For this review, take the finished solid that the model builds, in its own axes (mm). A direction names the side the tool comes from. Give positions to 0.01 mm unless a question says otherwise; leave off trailing zeros. Loops run counter-clockwise (first coordinate to the right, second up) from the corner with the lowest first, then second, coordinate; pieces in that order, holes last. Notation, with made-up numbers: M -1,-1 L 21,-1 A26 cw 21,25 Z; hole C -33,25 d2. An arc over 180 degrees is marked long. Use CSV: the item, a comma, the result in double quotes. Start each with the question number.
1. Take a section at D-D, the plane y = 19.5. Write out the cut boundary in (x, z), and give its area (3 significant figures).
2. The part is to be moulded in two halves that separate along X. For faces 1 (the face through (-72.5, -30, 8)), 2 (the face through (-72.5, -24, 2)), 3 (the face through (-8, -22.5, 2)), 4 (the face through (-215, 25, 6)), say which applies: pulls with the +X half, pulls with the -X half, needs draft (parallel to the pull), parting line crosses it, or undercut.
3. Take a section at A-A, the plane x = -7.5. Write out the cut boundary in (y, z).
4. Take a section at C-C, the plane x = -180. Write out the cut boundary in (y, z).
5. Tool access review of faces 5 (the face through (-72.5, -24, 13)), 6 (the face through (-72.5, 36, 2)), 7 (the face through (-65, -22.5, 2)), 8 (the face through (-63, -28, 10)): name each direction out of +Z, -Z, +X, -X, +Y, -Y from which nothing blocks a thin tool from reaching the whole face with its end or side.
6. To check wall thickness, follow line 1 (X direction, y = 30, z = 13.55); line 2 (Y direction, x = -65, z = 1.15); line 3 (Z direction, x = -59, y = 28). State the ranges of each line that lie inside material, in increasing order. Write a range as [from, to].
7. Take a section at B-B, the plane x = -65. State how many separate pieces and enclosed holes the cut face has, and give its area (3 significant figures).
8. Insertion check: P1, Ø4, axis at y = -26, z = 13.5, coming from the -X side; P2, Ø2, axis at y = 21, z = 4.5, coming from the -X side; P3, Ø3, axis at x = -107, z = 11, coming from the -Y side; P4, Ø3, axis at x = -7.5, y = -30, coming from the +Z side. Each pin has a flat end and moves straight along its axis. Give the tip position at first contact, or say it passes through.
from build123d import *

# Parameters (mm, degrees)
F1_DEPTH      = 15
F2_R          = 7.5
F3_DEPTH      = 240
F4_R          = 7.5
F5_DEPTH      = 30
F5_DEPTH_BACK = 30
F6_W          = 15
F6_H          = 15
F7_DEPTH      = 15
F9_DEPTH      = 40.1
F11_DEPTH     = 54.1
F12_R         = 2.5
F13_DEPTH     = 25
F15_R         = 2.5
F16_DEPTH     = 25
F17_R         = 7.5
F17_R_2       = 5
F18_DEPTH     = 25


with BuildPart() as f1:
    # F0 (on Top) → F1 (new body)
    with BuildSketch(Plane.XY):
        Polygon((-240, -22.5), (-240, -37.5), (0, -37.5), (0, -22.5), (-100, -22.5), (-100, 22.5), (0, 22.5), (0, 37.5), (-240, 37.5), (-240, 22.5), (-115, 22.5), (-115, -22.5), align=None)
    extrude(amount=F1_DEPTH)

    # F2 (on Right) → F3 (intersect)
    with BuildSketch(Plane.YZ):
        with Locations((-30, 7.5)):
            Circle(F2_R)
        with Locations((30, 7.5)):
            Circle(F2_R)
    extrude(amount=-F3_DEPTH, mode=Mode.INTERSECT)

    # F4 (on Front) → F5 (join, two sides)
    with BuildSketch(Plane.XZ) as f5_sk:
        with Locations((-100, 7.5)):
            Circle(F4_R)
    extrude(amount=F5_DEPTH)
    extrude(f5_sk.sketch, amount=-F5_DEPTH_BACK)

    # F6 (on Top) → F7 (join)
    with BuildSketch(Plane.XY):
        with Locations((-65, 30)):
            Rectangle(F6_W, F6_H)
        with Locations((-65, -30)):
            Rectangle(F6_W, F6_H)
        with Locations((-7.5, 30)):
            Rectangle(F6_W, F6_H)
        with Locations((-7.5, -30)):
            Rectangle(F6_W, F6_H)
    extrude(amount=F7_DEPTH)

    # F8 (on Front) → F9 (cut)
    with BuildSketch(Plane.XZ):
        Polygon((0, 0), (0, 10), (-72.5, 10), (-72.5, 5), (-57.5, 5), (-57.5, 0), align=None)
    extrude(amount=-F9_DEPTH, mode=Mode.SUBTRACT)

    # F10 (on Front) → F11 (cut)
    with BuildSketch(Plane.XZ):
        Polygon((0, 5), (0, 15), (-57.5, 15), (-57.5, 10), (-72.5, 10), (-72.5, 5), (-57.5, 5), align=None)
    extrude(amount=F11_DEPTH, mode=Mode.SUBTRACT)

    # F12 (on Top) → F13 (cut)
    with BuildSketch(Plane.XY):
        with Locations((-65, 30)):
            Circle(F12_R)
        with Locations((-65, -30)):
            Circle(F12_R)
        with Locations((-7.5, -30)):
            Circle(F12_R)
        with Locations((-7.5, 30)):
            Circle(F12_R)
    extrude(amount=F13_DEPTH, mode=Mode.SUBTRACT)

    # F15 (on offset) → F16 (cut)
    with BuildSketch(Plane(origin=(-240, 0, 0), x_dir=(0, -1, 0), z_dir=(-1, 0, 0))):
        with Locations((30, 7.5)):
            Circle(F15_R)
        with Locations((-30, 7.5)):
            Circle(F15_R)
    extrude(amount=-F16_DEPTH, mode=Mode.SUBTRACT)

    # F17 (on offset) → F18 (cut)
    with BuildSketch(Plane(origin=(-240, 0, 0), x_dir=(0, -1, 0), z_dir=(-1, 0, 0))):
        with Locations((30, 7.5)):
            Circle(F17_R)
        with Locations((30, 7.5)):
            Circle(F17_R_2, mode=Mode.SUBTRACT)
        with Locations((-30, 7.5)):
            Circle(F17_R)
        with Locations((-30, 7.5)):
            Circle(F17_R_2, mode=Mode.SUBTRACT)
    extrude(amount=-F18_DEPTH, mode=Mode.SUBTRACT)


solid = f1.part
Result set:
1,outline,"C -100,7.5 d15"
1,area,"177 mm2"
2,face 1,"pulls with the +X half"
2,face 2,"undercut"
2,face 3,"needs draft"
2,face 4,"pulls with the -X half"
3,outline,"M -37.5,0 L -32.5,0 L -32.5,5 L -37.5,5 Z; M -27.5,0 L -22.5,0 L -22.5,5 L -27.5,5 Z; M 22.5,10 L 27.5,10 L 27.5,15 L 22.5,15 Z; M 32.5,10 L 37.5,10 L 37.5,15 L 32.5,15 Z"
4,outline,"C -30,7.5 d15; C 30,7.5 d15"
5,face 5,"+Z"
5,face 6,"-Z, -X, +Y"
5,face 7,"+Z, -Z, +X"
5,face 8,"+X, +Y, -Y"
6,line 1,"[-215, -67.5], [-62.5, -10], [-5, 0]"
6,line 2,"[-37.5, -32.5], [-27.5, -22.5], [22.5, 27.5], [32.5, 37.5]"
6,line 3,"[0, 5], [10, 15]"
7,separate pieces,"8"
7,enclosed holes,"0"
7,area,"200 mm2"
8,P1,"x = -215"
8,P2,"x = -107.23"
8,P3,"y = -37.23"
8,P4,"through"
